Model file for the job. Use its own axes, mm. A direction names the side the tool comes from. Give positions to 0.01 mm unless a question says otherwise; leave off trailing zeros. Write each loop counter-clockwise with the first axis right and the second up, starting at its lowest first coordinate (ties: lowest second). Pieces come first, ordered by that corner, then holes. Notation, with made-up numbers: M 89,87.5 L 115,87.5 A19 cw 115,120.5 Z; hole C 5.5,30.5 d4. An arc over 180 degrees is marked long. Answer as a JSON object with one key per item and string values. Group by question number.
```python
from build123d import *

# Parameters (mm, degrees)
F0_R     = 12.5
F1_DEPTH = 20
F3_R     = 12.5
F4_DEPTH = 10
F5_W     = 25
F5_H     = 50
F6_DEPTH = 20


with BuildPart() as f1:
    # F0 (on Front) → F1 (new body)
    with BuildSketch(Plane.XZ):
        with BuildLine():
            Line((-50, -25), (0, -25))
            ThreePointArc((0, -25), (25, 0), (0, 25))
            Line((0, 25), (-50, 25))
            Line((-50, 25), (-50, -25))
        make_face()
        Circle(F0_R, mode=Mode.SUBTRACT)
    extrude(amount=F1_DEPTH)



with BuildPart() as f4:
    # F3 (on offset) → F4 (new body)
    with BuildSketch(Plane.XZ.offset(40)):
        with BuildLine():
            Line((0, 25), (-50, 25))
            Line((-50, 25), (-50, -25))
            Line((-50, -25), (0, -25))
            ThreePointArc((0, -25), (25, 0), (0, 25))
        make_face()
        Circle(F3_R, mode=Mode.SUBTRACT)
    extrude(amount=F4_DEPTH)


with BuildPart() as f1_1:
    add(f1.part)

    add(f4.part)  # F6 merges F4
    # F5 (on face) → F6 (join, through all)
    with BuildSketch(Plane.XZ.offset(20)):
        with Locations((-37.5, 0)):
            Rectangle(F5_W, F5_H)
    extrude(amount=F6_DEPTH)


solid = f1_1.part
```
Q1. Slice it at B-B, the plane z = 0. Write the cut outline in (x, y), then the cut area to 3 significant figures.
Q2. Slice it at D-D, the plane z = 10. Write the cut outline in (x, y), then the cut area to 3 significant figures.
Q3. Drop flat-ended pins along their axis: P1, Ø10, axis at y = -41, z = 5, coming from the +X side; P2, Ø25, axis at x = -5, z = 7.5, coming from the +Y side; P3, Ø4, axis at x = 16.5, y = -9.5, coming from the -Z side; P4, Ø6, axis at x = -13.5, y = -24, coming from the +Z side. Give the stop position or say it passes through.
Q4. Wall check: L1, parallel to Y at x = -20, z = -6.5; L2, parallel to X at y = -29, z = -2.5; L3, parallel to Z at x = 2, y = -11.5. Give the ranges that are in metal, low to high.
Q5. Slice it at A-A, the plane x = -11. Write the cut outline in (y, z), then the cut area to 3 significant figures.
Q6. 3-axis set-ups, long thin cutter, end or side, ignore diameter. For faces 1 (the flat face through (-25.3, -24.6, -25)), 2 (the flat face through (-11.5, -40, 5.9)): which of +Z, -Z, +X, -X, +Y, -Y reach the whole face in a straight line?
Q7. Slice it at C-C, the plane y = -13.5. Write the cut outline in (x, z), then the cut area to 3 significant figures.
Q8. Two-plate mould, pull along Y, no slides. Class faces 3 (the cylindrical face through (24.994, -44.93, -0.55)), 4 (the flat face through (-21, 0, 0)), 5 (the flat face through (-25, -30, 0)): +Y half, -Y half, draft (parallel to the pull), parting line (faces both ways), or undercut.
Solved:
{
 "1": {"outline": "M -50,-50 L -12.5,-50 L -12.5,-40 L -25,-40 L -25,-20 L -12.5,-20 L -12.5,0 L -50,0 Z; M 12.5,-50 L 25,-50 L 25,-40 L 12.5,-40 Z; M 12.5,-20 L 25,-20 L 25,0 L 12.5,0 Z", "area": "2,000 mm²"},
 "2": {"outline": "M -50,-50 L -7.5,-50 L -7.5,-40 L -25,-40 L -25,-20 L -7.5,-20 L -7.5,0 L -50,0 Z; M 7.5,-50 L 22.91,-50 L 22.91,-40 L 7.5,-40 Z; M 7.5,-20 L 22.91,-20 L 22.91,0 L 7.5,0 Z", "area": "2,240 mm²"},
 "3": {"P1": "stops at x = 25", "P2": "stops at y = 0", "P3": "stops at z = -20.37", "P4": "passes through"},
 "4": {"L1": "y = -50 to -40, -20 to 0", "L2": "x = -50 to -25", "L3": "z = -24.92 to -12.34, 12.34 to 24.92"},
 "5": {"outline": "M -50,-25 L -40,-25 L -40,-5.94 L -50,-5.94 Z; M -50,5.94 L -40,5.94 L -40,25 L -50,25 Z; M -20,-25 L 0,-25 L 0,-5.94 L -20,-5.94 Z; M -20,5.94 L 0,5.94 L 0,25 L -20,25 Z", "area": "1,140 mm²"},
 "6": {"face 1": "-Z, +X, -X, +Y, -Y", "face 2": "+Z, -Z, +X"},
 "7": {"outline": "M -50,-25 L 0,-25 A25 ccw 0,25 L -50,25 Z; hole C 0,0 d25", "area": "2,990 mm²"},
 "8": {"face 3": "draft", "face 4": "+Y half", "face 5": "undercut"}
}
